Input: part model. Units: mm. Frame: model coordinates. A direction names the side the tool comes from. Round coordinates to 2 decimals unless told otherwise and drop trailing zeros. Loops run counter-clockwise (first coordinate to the right, second up) from the corner with the lowest first, then second, coordinate; pieces in that order, holes last. Notation, with made-up numbers: (35, 8.25) - (64, 8.25) arc R14 ccw to (64, 35.25) - close; hole circle Ø9 at (62.5, 48). An arc over 180 degrees is marked (long way). Use CSV: the item, a comma, the result in double quotes. Start each with the question number.
1. Cut plane D-D (z = -2.75). Return loops of the section in (x, y), and give its area (3 significant figures).
2. Cut plane A-A (x = 2.5). Return loops of the section in (y, z), and give its area (3 significant figures).
3. Access query for faces 4 (the flat face through (8, 27.233, 11)), 5 (the flat face through (8, 0, -5)). Directions: +Z, -Z, +X, -X, +Y, -Y. A direction counts if a zero-diameter tool reaches every point of the face in a straight line with its end or side. Return the directions, or none.
4. Pull-direction query (Y, two-part tool) for faces 1 (the flat face through (54.941, 0, 11)), 2 (the flat face through (59.941, 0, 10)), 3 (the cylindrical face through (58.438, -30.816, 10.14)); classes: +Y half, -Y half, draft (parallel to the pull), parting line (faces both ways), or undercut.
5. Pin query (flat end, axial travel): P1, Ø5, axis at y = 4, z = 16, coming from the -X side; P2, Ø5, axis at x = -22, y = -5, coming from the +Z side; P3, Ø1.5, axis at y = 22, z = -1, coming from the +X side. Return the tip coordinate at first contact, or that it passes through.
6. Cut plane C-C (z = 12.25). Return loops of the section in (x, y), and give its area (3 significant figures).
7. Material intervals for probe 1 along Y at (x, z) = (-23, 8.5); probe 2 along Z at (x, y) = (17.5, 27.5); probe 3 along Z at (x, y) = (-7, 25), sorted ascending. Write a range as from..to.
8. Cut plane B-B (y = -1). Return loops of the section in (x, z), and give its area (3 significant figures).
```python
from build123d import *

# Parameters (mm, degrees)
SKETCH_W          = 92.858264
SKETCH_H          = 54.475084
PAD_DEPTH         = 20
THICKNESS_T       = 5
THICKNESS_FACE4_W = 54.475084
THICKNESS_FACE4_H = 92.858264
PAD001_DEPTH      = 2


with BuildPart() as part:
    # Sketch → Pad (new body)
    with BuildSketch(Plane.XY):
        with Locations((8.511961, -0.004594)):
            Rectangle(SKETCH_W, SKETCH_H)
    extrude(amount=PAD_DEPTH)

    # Thickness
    thickness_openings = [part.faces().sort_by_distance(p)[0] for p in [
        (8.511961, -0.004594, 20),
        (-37.917171, -0.004594, 10),
    ]]
    offset(amount=THICKNESS_T, openings=thickness_openings)

    # Thickness Face4 → Pad001 (add)
    with BuildSketch(Plane(origin=(8.511961, -0.004594, 0), x_dir=(0, 1, 0), z_dir=(0, 0, 1))):
        Rectangle(THICKNESS_FACE4_W, THICKNESS_FACE4_H)
    extrude(amount=PAD001_DEPTH)


solid = part.part
```
Established:
1,outline,"(-37.92, -31.42) - (54.94, -31.42) arc R4.18 ccw to (59.12, -27.24) - (59.12, 27.23) arc R4.18 ccw to (54.94, 31.41) - (-37.92, 31.41) - close"
1,area,"6,090 mm2"
2,outline,"(-32.24, 0) arc R5 ccw to (-27.24, -5) - (27.23, -5) arc R5 ccw to (32.23, 0) - (32.23, 20) - (27.23, 20) - (27.23, 2) - (-27.24, 2) - (-27.24, 20) - (-32.24, 20) - close"
2,area,"621 mm2"
3,face 4,"+Z, -X"
3,face 5,"-Z, +X, -X, +Y, -Y"
4,face 1,"undercut"
4,face 2,"draft"
4,face 3,"-Y half"
5,P1,"stops at x = 54.94"
5,P2,"stops at z = 2"
5,P3,"stops at x = 59.93"
6,outline,"(-37.92, -32.24) - (54.94, -32.24) arc R5 ccw to (59.94, -27.24) - (59.94, 27.23) arc R5 ccw to (54.94, 32.23) - (-37.92, 32.23) - (-37.92, 27.23) - (54.94, 27.23) - (54.94, -27.24) - (-37.92, -27.24) - close"
6,area,"1,240 mm2"
7,probe 1,"y = -32.24..-27.24, 27.23..32.23"
7,probe 2,"z = -4.99..20"
7,probe 3,"z = -5..2"
8,outline,"(-37.92, -5) - (54.94, -5) arc R5 ccw to (59.94, 0) - (59.94, 20) - (54.94, 20) - (54.94, 2) - (-37.92, 2) - close"
8,area,"770 mm2"
